Job drawing, mm, ordinate dimensions from the low corner. One solid piece. A direction names the side the tool comes from. Give positions to 0.01 mm unless a question says otherwise; leave off trailing zeros. Write each loop counter-clockwise with the first axis right and the second up, starting at its lowest first coordinate (ties: lowest second). Pieces come first, ordered by that corner, then holes. Notation, with made-up numbers: (83, -14) - (121, -14) arc R8 ccw to (121, -7) - close; hole circle Ø2 at (9.25, 81.5). An arc over 180 degrees is marked (long way). Put each result on its own line as item: value. Start each with the question number.
1. Cut at A-A on x = 51.5. List the corners of the cut face in (y, z), and give its area (3 significant figures).
2. Cut at B-B on y = 68. List the corners of the cut face in (x, z), and give its area (3 significant figures).
3. Mould opens along X. For the marked faces 1, 2 and 3 say: +X half, -X half, draft (parallel to the pull), parting line (faces both ways), or undercut.
4. Cut at C-C on z = 61. List the corners of the cut face in (x, y) (3 decimals), and give its area (3 significant figures).
5. Tool access for the marked faces 4 and 5: list every direction of +Z, -Z, +X, -X, +Y, -Y with a clear straight run to the whole face (end or side of a thin tool).
6. Cut at D-D on x = 17.5. List the corners of the cut face in (y, z), and give its area (3 significant figures).
7. Wall check: line 1 (Y direction, x = 50, z = 61.5); line 2 (Z direction, x = 31.5, y = 29); line 3 (Z direction, x = 89.5, y = 21.5). Give the ranges that are in metal, low to high.
8. Drop flat-ended pins along their axis: pin 1 (4 mm diameter, centred on x = 43, y = 31.5, fed in from -Z); pin 2 (8 mm diameter, centred on x = 44, y = 68, fed in from +Z). Give the stop position or say it passes through.
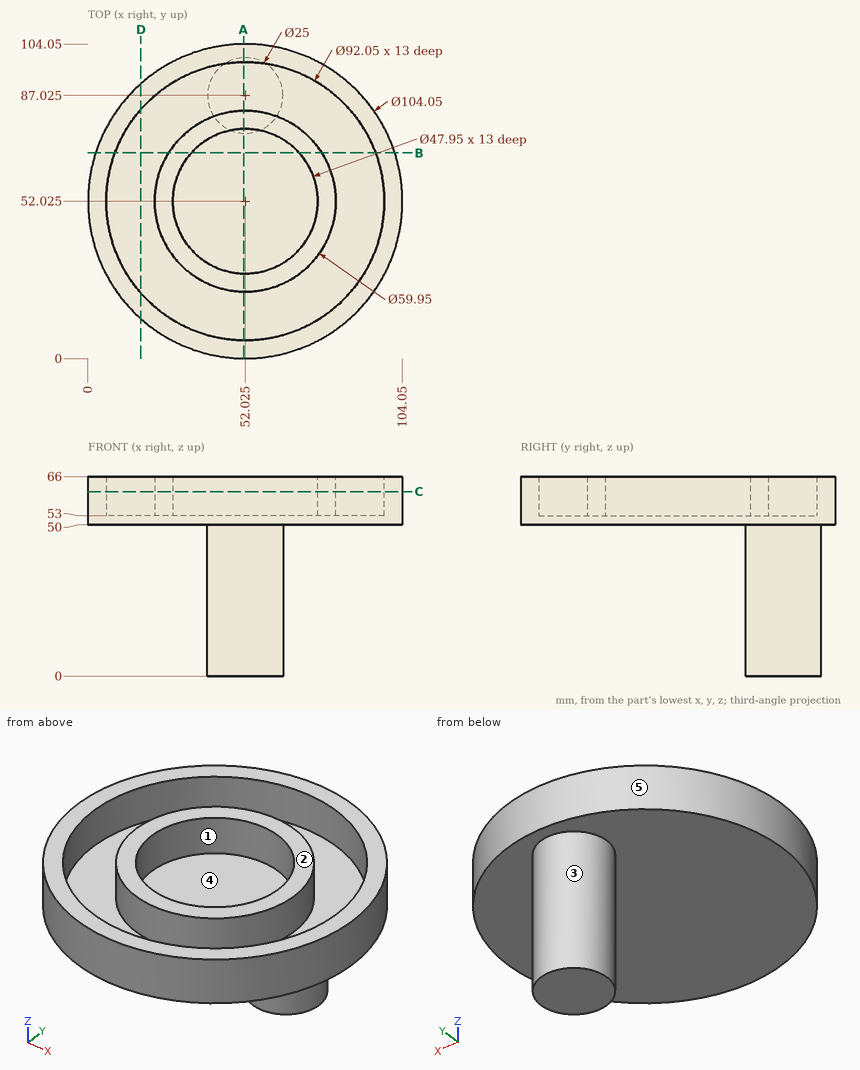
Report:
1. outline: (0, 50) - (74.54, 50) - (74.54, 0) - (99.51, 0) - (99.51, 50) - (104.05, 50) - (104.05, 66) - (98.05, 66) - (98.05, 53) - (82, 53) - (82, 66) - (75.99, 66) - (75.99, 53) - (28.06, 53) - (28.06, 66) - (22.05, 66) - (22.05, 53) - (6, 53) - (6, 66) - (0, 66) - close
1. area: 1,870 mm²
2. outline: (2.51, 50) - (101.54, 50) - (101.54, 66) - (95.19, 66) - (95.19, 53) - (77.39, 53) - (77.39, 66) - (69.9, 66) - (69.9, 53) - (34.15, 53) - (34.15, 66) - (26.66, 66) - (26.66, 53) - (8.86, 53) - (8.86, 66) - (2.51, 66) - close
2. area: 657 mm²
3. face 1: undercut
3. face 2: draft
3. face 3: parting line
4. outline: circle Ø104.05 at (52.025, 52.025); circle Ø59.95 at (52.025, 52.025); hole circle Ø92.05 at (52.025, 52.025); hole circle Ø47.95 at (52.025, 52.025)
4. area: 2,870 mm²
5. face 4: +Z
5. face 5: +Z, -Z
6. outline: (13.11, 50) - (90.94, 50) - (90.94, 66) - (82.46, 66) - (82.46, 53) - (21.59, 53) - (21.59, 66) - (13.11, 66) - close
6. area: 454 mm²
7. line 1: y = 0.04 to 6.04, 22.12 to 28.14, 75.91 to 81.93, 98.01 to 104.01
7. line 2: z = 50 to 53
7. line 3: z = 50 to 66
8. pin 1: stops at z = 50
8. pin 2: stops at z = 53
